Can you work these out from the model? Positions are in its coordinate system, mm. Give positions to 0.01 mm unless a question says otherwise; leave off trailing zeros. Order: outer loops, then holes, each group sorted by start corner. A loop starts at its lowest first (then second) coordinate and runs counter-clockwise, first axis right, second up.
Item 1: I want a section at B-B, the plane y = -42. Write out the boundary of the cut face in (x, z), then the cut area to 3 significant figures.
Item 2: I want a section at C-C, the plane z = 0.6. Write out the boundary of the cut face in (x, y).
Item 3: I'm going to push flat-ended pins straight in: pin 1 Ø0.8 at (x, z) = (-109.5, 1) entering from -Y; pin 2 Ø0.8 at (x, z) = (291, 1) entering from -Y. Where does each tip first touch, or does it pass through?
Item 4: If I drill on line 1 along X through (y, z) = (2, 0.75); line 2 along X through (y, z) = (-70, 0.8); line 3 along Y through (x, z) = (-253.5, 0.9), over which ranges is the centre line in solid material (lowest first)?
Item 5: I want a section at A-A, the plane y = 56.5. Write out the boundary of the cut face in (x, z).
Item 6: I want a section at D-D, the plane x = 51. Write out the boundary of the cut face in (y, z).
Autodesk Inventor part; units mm, degrees
ref_plane "YZ Plane" through (0, 0, 0) normal (1, 0, 0) x (0, 1, 0)
ref_plane "XZ Plane" through (0, 0, 0) normal (0, 1, 0) x (-1, 0, 0)
ref_plane "XY Plane" through (0, 0, 0) normal (0, 0, 1) x (1, 0, 0)
sketch "Sketch1" plane through (0, 0, 0) normal (0, 0, 1) x (1, 0, 0)
  line L0 (-368.3, -177.8) -> (368.3, -177.8)
  line L1 (368.3, -177.8) -> (368.3, 177.8)
  line L2 (368.3, 177.8) -> (-368.3, 177.8)
  line L3 (-368.3, 177.8) -> (-368.3, -177.8)
  line L4 (-368.3, -177.8) -> (368.3, 177.8) construction
  line L5 (368.3, -177.8) -> (-368.3, 177.8) construction
  point P0 (0, 0)
  dimension "d0" = 355.6
  dimension "d1" = 736.6
extrude "Extrusion1" add sketch "Sketch1" along normal blind 1.5875
sketch "Sketch2" plane through (0, 0, 1.5875) normal (0, 0, 1) x (1, 0, 0)
  line L0 (-368.3, -177.8) -> (368.3, -177.8)
  line L1 (368.3, -177.8) -> (368.3, 177.8)
  line L2 (368.3, 177.8) -> (-368.3, 177.8)
  line L3 (-368.3, 177.8) -> (-368.3, -177.8)
  line L4 (-368.3, -177.8) -> (368.3, -177.8)
  line L5 (-342.9, -177.8) -> (-266.7, -177.8)
  line L6 (-266.7, -177.8) -> (-266.7, 127)
  line L7 (-266.7, 127) -> (-342.9, 127)
  line L8 (-342.9, 127) -> (-342.9, -177.8)
  point P0 (0, 0)
  dimension "d4" = 50.8
  dimension "d5" = 76.2
  dimension "d6" = 25.4
extrude "Extrusion2" cut sketch "Sketch2" against normal through all contours L8 L7 L6 L0
mirror "Mirror1" about plane through (0, 0, 0) normal (1, 0, 0) of "Extrusion2"
sketch "Sketch3" plane through (0, 0, 1.5875) normal (0, 0, 1) x (1, 0, 0)
  line L0 (342.9, 127) -> (342.9, -177.8)
  line L1 (342.9, -177.8) -> (368.3, -177.8)
  line L2 (368.3, -177.8) -> (368.3, 177.8)
  line L3 (368.3, 177.8) -> (-368.3, 177.8)
  line L4 (-368.3, 177.8) -> (-368.3, -177.8)
  line L5 (-368.3, -177.8) -> (-342.9, -177.8)
  line L6 (-342.9, -177.8) -> (-342.9, 127)
  line L7 (-342.9, 127) -> (-266.7, 127)
  line L8 (-266.7, 127) -> (-266.7, -177.8)
  line L9 (-266.7, -177.8) -> (266.7, -177.8)
  line L10 (266.7, -177.8) -> (266.7, 127)
  line L11 (266.7, 127) -> (342.9, 127)
  line L12 (-266.7, -177.8) -> (266.7, -177.8)
  line L13 (266.7, -177.8) -> (266.7, -25.4)
  line L14 (266.7, -25.4) -> (-266.7, -25.4)
  line L15 (-266.7, -25.4) -> (-266.7, -177.8)
  point P0 (0, 0)
  dimension "d9" = 152.4
extrude "Extrusion3" cut sketch "Sketch3" against normal through all contours L10 L9 L8 L14
properties part number "Human Player Ramp Panel" material "Polycarbonate, Clear"
Results list:
1. outline: (-368.3, 0) - (-342.9, 0) - (-342.9, 1.59) - (-368.3, 1.59) - close; (342.9, 0) - (368.3, 0) - (368.3, 1.59) - (342.9, 1.59) - close
1. area: 80.6 mm2
2. outline: (-368.3, -177.8) - (-342.9, -177.8) - (-342.9, 127) - (-266.7, 127) - (-266.7, -25.4) - (266.7, -25.4) - (266.7, 127) - (342.9, 127) - (342.9, -177.8) - (368.3, -177.8) - (368.3, 177.8) - (-368.3, 177.8) - close
3. pin 1: stops at y = -25.4
3. pin 2: stops at y = 127
4. line 1: x = -368.3 to -342.9, -266.7 to 266.7, 342.9 to 368.3
4. line 2: x = -368.3 to -342.9, 342.9 to 368.3
4. line 3: y = -25.4 to 177.8
5. outline: (-368.3, 0) - (-342.9, 0) - (-342.9, 1.59) - (-368.3, 1.59) - close; (-266.7, 0) - (266.7, 0) - (266.7, 1.59) - (-266.7, 1.59) - close; (342.9, 0) - (368.3, 0) - (368.3, 1.59) - (342.9, 1.59) - close
6. outline: (-25.4, 0) - (177.8, 0) - (177.8, 1.59) - (-25.4, 1.59) - close
